Input: dimensioned drawing with shaded views. Units: mm. Origin: part minimum x, y, z. A direction names the side the tool comes from. Coordinates: 2 decimals unless noted, no trailing zeros. Loops run counter-clockwise (first coordinate to the right, second up) from the corner with the lowest first, then second, coordinate; pieces in that order, holes last.
Item 1: Reachability of the marked faces 1 and 2 from +Z, -Z, +X, -X, +Y, -Y: full face, straight path, thin tool, end or side. Return the list, or none.
Item 2: Pull-direction query (X, two-part tool) for the marked faces 3, 4 and 5; classes: released by +X, released by -X, zero draft, split by the parting line, or undercut.
Item 3: Section D-D on y = 38.5. Return loops of the section in (x, z).
Item 4: Section B-B on x = 12. Return loops of the section in (y, z).
Item 5: Ray query, line 1 along Z through (x, y) = (35.5, 16); line 2 along X through (y, z) = (49, 5.5); line 3 along X through (y, z) = (11, 21). Return the intervals inside material, ascending.
Item 6: Section A-A on z = 8.25. Return loops of the section in (x, y) (1 decimal), and give its area (3 significant figures).
Item 7: Section C-C on z = 16. Return loops of the section in (x, y) (1 decimal).
Item 8: Contact query for flat-ended pins moving along their axis: P1, Ø21, axis at x = 12.5, y = 25, coming from the -Z side; P2, Ø2.5, axis at x = 45.14, y = 47.69, coming from the -Z side; P3, Ø2.5, axis at x = 44.5, y = 48.5, coming from the +Z side; P4, Ø8, axis at x = 11, z = 14.5, coming from the -Y side. Output: stop coordinate, or through.
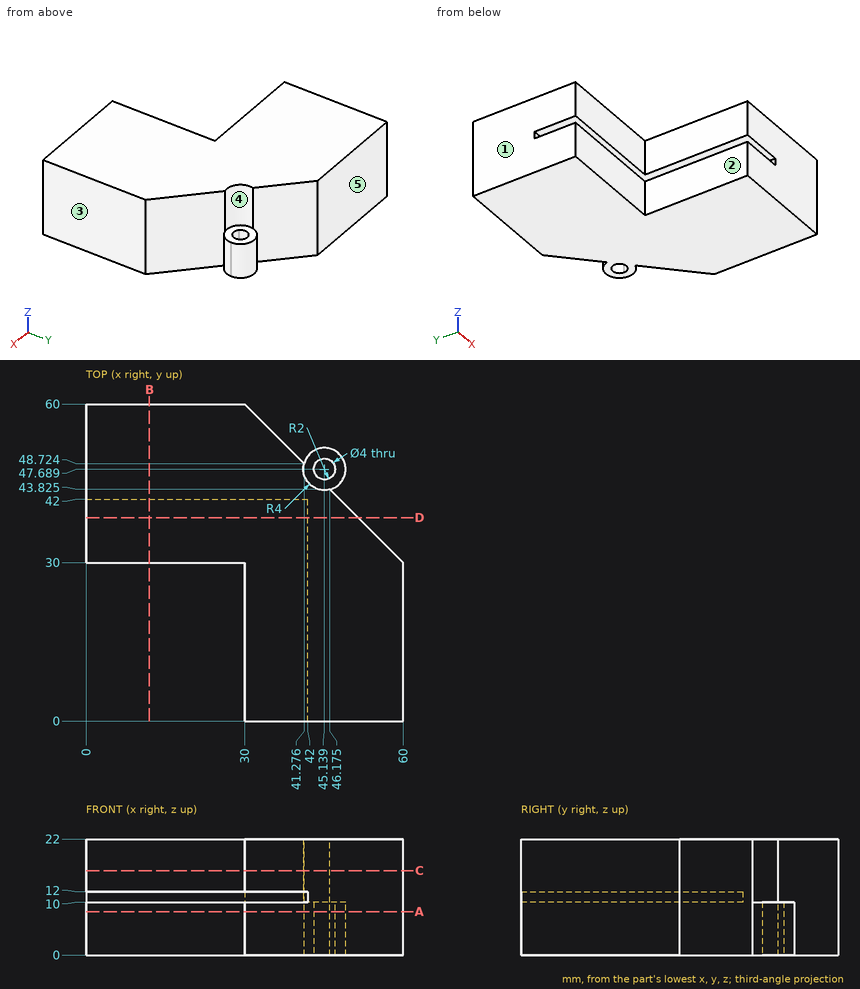
Results found:
1. face 1: +Z, -Z, -X, +Y, -Y
1. face 2: +Z, -Z, -X, -Y
2. face 3: released by +X
2. face 4: undercut
2. face 5: zero draft
3. outline: (0, 0) - (51.5, 0) - (51.5, 22) - (0, 22) - (0, 12) - (42, 12) - (42, 10) - (0, 10) - close
4. outline: (30, 0) - (60, 0) - (60, 22) - (30, 22) - (30, 12) - (42, 12) - (42, 10) - (30, 10) - close
5. line 1: z = 0 to 10, 12 to 22
5. line 2: x = 0 to 41, 41.36 to 43.63, 46.65 to 48.92
5. line 3: x = 30 to 60
6. outline: (0, 30) - (30, 30) - (30, 0) - (60, 0) - (60, 30) - (46.2, 43.8) arc R4 ccw (long way) to (41.3, 48.7) - (30, 60) - (0, 60) - close; hole circle Ø4 at (45.1, 47.7)
6. area: 2,280 mm2
7. outline: (0, 30) - (30, 30) - (30, 0) - (60, 0) - (60, 30) - (46.2, 43.8) arc R4 cw to (41.3, 48.7) - (30, 60) - (0, 60) - close
8. P1: stops at z = 0
8. P2: passes through
8. P3: stops at z = 10
8. P4: stops at y = 30
